```python
from build123d import *

# Parameters (mm, degrees)
BOSS_EXTRUDE2_DEPTH = 5
SKETCH3_R           = 1.7
CUT_EXTRUDE1_DEPTH  = 5


with BuildPart() as part:
    # Sketch1 → Boss-Extrude2 (new body)
    with BuildSketch(Plane.XY):
        with BuildLine():
            Line((-65, -20), (-65, -33))
            ThreePointArc((-65, -33), (-62.071067812, -40.071067812), (-55, -43))
            Line((-55, -43), (55, -43))
            ThreePointArc((55, -43), (62.071067812, -40.071067812), (65, -33))
            Line((65, -33), (65, -20))
            Line((65, -20), (69.5, -20))
            ThreePointArc((69.5, -20), (76.571067812, -17.071067812), (79.5, -10))
            Line((79.5, -10), (79.5, 10))
            ThreePointArc((79.5, 10), (76.571067812, 17.071067812), (69.5, 20))
            Line((69.5, 20), (65, 20))
            Line((65, 20), (65, 33))
            ThreePointArc((65, 33), (62.071067812, 40.071067812), (55, 43))
            Line((55, 43), (-55, 43))
            ThreePointArc((-55, 43), (-62.071067812, 40.071067812), (-65, 33))
            Line((-65, 33), (-65, 20))
            Line((-65, 20), (-69.5, 20))
            ThreePointArc((-69.5, 20), (-76.571067812, 17.071067812), (-79.5, 10))
            Line((-79.5, 10), (-79.5, -10))
            ThreePointArc((-79.5, -10), (-76.571067812, -17.071067812), (-69.5, -20))
            Line((-69.5, -20), (-65, -20))
        make_face()
    extrude(amount=BOSS_EXTRUDE2_DEPTH)

    # Sketch3 → Cut-Extrude1 (cut)
    with BuildSketch(Plane.XY.offset(5)):
        with Locations((-47.5, -15)):
            Circle(SKETCH3_R)
        with Locations((-47.5, 15)):
            Circle(SKETCH3_R)
        with Locations((72.5, 15)):
            Circle(SKETCH3_R)
        with Locations((47.52365162, 15)):
            Circle(SKETCH3_R)
        with Locations((72.5, -15)):
            Circle(SKETCH3_R)
        with Locations((47.5, -15)):
            Circle(SKETCH3_R)
        with BuildLine():
            Line((15, 38), (-15, 38))
            ThreePointArc((-15, 38), (-20, 33), (-15, 28))
            Line((-15, 28), (15, 28))
            ThreePointArc((15, 28), (20, 33), (15, 38))
        make_face()
        with BuildLine():
            Line((15, -28), (-15, -28))
            ThreePointArc((-15, -28), (-20, -33), (-15, -38))
            Line((-15, -38), (15, -38))
            ThreePointArc((15, -38), (20, -33), (15, -28))
        make_face()
        with Locations((-72.5, -15)):
            Circle(SKETCH3_R)
        with Locations((-72.5, 15)):
            Circle(SKETCH3_R)
        with Locations((-26.692902898, 21.354322319)):
            Circle(SKETCH3_R)
        with Locations((-26.692902898, 1.354322319)):
            Circle(SKETCH3_R)
        with Locations((-26.692902898, -18.645677681)):
            Circle(SKETCH3_R)
        with Locations((28.307097102, -18.645677681)):
            Circle(SKETCH3_R)
        with Locations((28.307097102, 1.354322319)):
            Circle(SKETCH3_R)
        with Locations((28.307097102, 21.354322319)):
            Circle(SKETCH3_R)
        with Locations((-52, 23)):
            Circle(SKETCH3_R)
        with Locations((-52, -23)):
            Circle(SKETCH3_R)
        with Locations((52, -23)):
            Circle(SKETCH3_R)
        with Locations((52, 23)):
            Circle(SKETCH3_R)
    extrude(amount=-CUT_EXTRUDE1_DEPTH, mode=Mode.SUBTRACT)


solid = part.part
```
Source: CAD feature listing. Evaluate the final solid. Frame: model axes, mm. A direction names the side the tool comes from. Coordinates: 2 decimals unless noted, no trailing zeros. Loops run counter-clockwise (first coordinate to the right, second up) from the corner with the lowest first, then second, coordinate; pieces in that order, holes last. Notation, with made-up numbers: M 29.5,65.25 L 58.5,65.25 A9 cw 58.5,81.25 Z; hole C -22,75 d10. An arc over 180 degrees is marked long. Use CSV: the item, a comma, the result in double quotes.
(1) Cut plane A-A on x = 7.5. Return loops of the section in (y, z), and give its area (3 significant figures).
Answers follow:
outline,"M -43,0 L -38,0 L -38,5 L -43,5 Z; M -28,0 L 28,0 L 28,5 L -28,5 Z; M 38,0 L 43,0 L 43,5 L 38,5 Z"
area,"330 mm²"
(2) Line query: line 1 (Y direction, x = 9, z = 1.45); line 2 (Y direction, x = -26.5, z = 0.5); line 3 (Y direction, x = 16, z = 2.8). Output: solid intervals per line, ascending. Write a range as [from, to].
Answers follow:
line 1,"[-43, -38], [-28, 28], [38, 43]"
line 2,"[-43, -20.33], [-16.96, -0.33], [3.04, 19.67], [23.04, 43]"
line 3,"[-43, -37.9], [-28.1, 28.1], [37.9, 43]"
(3) Cut plane B-B on y = -35.5. Return loops of the section in (x, z).
Answers follow:
outline,"M -64.68,0 L -19.33,0 L -19.33,5 L -64.68,5 Z; M 19.33,0 L 64.68,0 L 64.68,5 L 19.33,5 Z"
(4) Reachability of faces 5 (the face through (-65, -26, 2)), 6 (the face through (65, 26, 2)), 7 (the face through (-20, 33, 3)) from +Z, -Z, +X, -X, +Y, -Y: full face, straight path, thin tool, end or side. Return the list, or none.
Answers follow:
face 5,"+Z, -Z, -X, -Y"
face 6,"+Z, -Z, +X, +Y"
face 7,"+Z, -Z"
(5) Draft query along X for faces 1 (the face through (-76.49, 17.15, 2.46)), 2 (the face through (-53.7, -22.93, 2.54)), 3 (the face through (62.15, 39.99, 2.46)), 4 (the face through (29.877, -19.297, 2.535)). Return one class per face: pulls with the +X half, pulls with the -X half, needs draft (parallel to the pull), parting line crosses it, or undercut.
Answers follow:
face 1,"pulls with the -X half"
face 2,"undercut"
face 3,"pulls with the +X half"
face 4,"undercut"
(6) Cut plane C-C on y = -23. Return loops of the section in (x, z).
Answers follow:
outline,"M -65,0 L -53.7,0 L -53.7,5 L -65,5 Z; M -50.3,0 L 50.3,0 L 50.3,5 L -50.3,5 Z; M 53.7,0 L 65,0 L 65,5 L 53.7,5 Z"
(7) Cut plane D-D on z = 2.75. Give the number of separate pieces and of enclosed holes in the cut face, and give its area (3 significant figures).
Answers follow:
separate pieces,"1"
enclosed holes,"20"
area,"11,200 mm²"
(8) Contact query for flat-ended pins moving along their axis: pin 1 (1.5 mm diameter, centred on y = 28.5, z = 3.5, fed in from +X); pin 2 (1.3 mm diameter, centred on x = -67, z = 2, fed in from -Y). Output: stop coordinate, or through.
Answers follow:
pin 1,"x = 65"
pin 2,"y = -20"
